Read the model definition and answer for the solid it produces. Units are mm, in the model's axes. A direction names the side the tool comes from. Coordinates: 2 decimals unless noted, no trailing zeros. Write each loop counter-clockwise with the first axis right and the second up, starting at its lowest first coordinate (ties: lowest second). Pieces come first, ordered by that corner, then holes.
1) The part is cut by section A-A (y = 15). Determine the outline of the cut face in (x, z).
2) Each of these flat-tipped pins is pushed along its axis until it touches: pin 1 Ø4 at (x, z) = (1.5, -83.5) entering from -Y; pin 2 Ø4 at (y, z) = (30.5, -4.5) entering from -X. Where does it stop, or does it pass through?
3) Which of the six approach directions +Z, -Z, +X, -X, +Y, -Y give full straight-line access (tool end or side, diameter ignored) to faces 1 (the face through (17, -1, -3)), 2 (the face through (7, 53.5, -3))?
4) Determine the mould class of faces 3 (the face through (15.5, 0, -3)), 4 (the face through (0, 1, -200)), 5 (the face through (0, 1, 200)) for opening direction Z: +Z half, -Z half, draft (parallel to the pull), parting line (faces both ways), or undercut.
5) Find the intervals of material crossed by line 1 (X direction, y = -35, z = 199.2); line 2 (Z direction, x = -2.5, y = 2.5); line 3 (X direction, y = -20, z = 199.2), in increasing order.
6) The part is cut by section B-B (z = 64.5). Determine the outline of the cut face in (x, y), then the cut area to 3 significant figures.
Autodesk Inventor part; units mm, degrees
ref_plane "YZ Plane" through (0, 0, 0) normal (1, 0, 0) x (0, 1, 0)
ref_plane "XZ Plane" through (0, 0, 0) normal (0, 1, 0) x (-1, 0, 0)
ref_plane "XY Plane" through (0, 0, 0) normal (0, 0, 1) x (1, 0, 0)
sketch "Skizze1" plane through (0, 0, 0) normal (0, 0, 1) x (1, 0, 0)
  line L0 (-17, -55) -> (17, -55)
  line L1 (17, -55) -> (17, 55)
  line L2 (17, 55) -> (-17, 55)
  line L3 (-17, 55) -> (-17, -55)
  line L4 (-17, 55) -> (17, -55) construction
  line L5 (-17, -55) -> (17, 55) construction
  point P0 (0, 0)
  point P1 (0, 0)
  dimension "d0" = 34
  dimension "d2" = 110
extrude "Extrusion1" add sketch "Skizze1" along normal mid plane 400
sketch "Skizze2" plane through (0, 0, 200) normal (0, 0, 1) x (1, 0, 0)
  line L0 (-17, -55) -> (17, -55)
  line L1 (17, -55) -> (17, 55)
  line L2 (17, 55) -> (-17, 55)
  point P0 (0, 0)
  point P1 (2, 30)
  point P2 (9, -20)
  point P3 (2, -35)
  dimension "d5" = 25
  dimension "d6" = 15
  dimension "d30" = 50
  dimension "d31" = 8
  dimension "d32" = 7
  dimension "d33" = 35
  dimension "d40" = 20
  dimension "d41" = 15
hole "Bohrung1" at (2, 30, 200) at (9, -20, 200) at (2, -35, 200) direction (0, 0, -1) diameter 4 end through all
sketch "Skizze4" plane through (-17, -55, 200) normal (-1, 0, 0) x (0, 0, 1)
  line L0 (0, 0) -> (-400, 0)
  line L1 (0, 110) -> (0, 0)
  line L2 (-400, 110) -> (0, 110)
  line L3 (-400, 0) -> (-400, 110)
  line L4 (-398.5, 108.5) -> (-1.5, 108.5)
  line L5 (-1.5, 108.5) -> (-1.5, 0)
  line L6 (-1.5, 0) -> (-398.5, 0)
  line L7 (-398.5, 0) -> (-398.5, 108.5)
  point P0 (-200, 55)
  dimension "d34" = 1.5
  dimension "d35" = 0
  dimension "d36" = 1.5
  dimension "d37" = 1.5
extrude "Extrusion2" cut sketch "Skizze4" against normal blind 32.5 contours L0 L7 L4 L5
sketch "Skizze5" plane through (-17, 55, 200) normal (0, 1, 0) x (1, 0, 0)
  line L0 (34, 0) -> (0, 0)
  line L1 (34, 400) -> (34, 0)
  line L2 (0, 400) -> (34, 400)
  line L3 (0, 398.5) -> (16, 398.5)
  line L4 (16, 398.5) -> (16, 1.5)
  line L5 (16, 1.5) -> (0, 1.5)
  line L6 (0, 1.5) -> (0, 398.5)
  point P0 (17, 200)
  dimension "d42" = 1.5
  dimension "d43" = 1.5
  dimension "d44" = 18
extrude "Extrusion3" cut sketch "Skizze5" against normal blind 32.5
properties part number "bewegliche achse horizontal" material "Stahl"
Reported:
1. outline: (-17, -200) - (17, -200) - (17, 200) - (-17, 200) - (-17, 198.5) - (15.5, 198.5) - (15.5, -198.5) - (-17, -198.5) - close
2. pin 1: stops at y = 53.5
2. pin 2: stops at x = 15.5
3. face 1: +Z, -Z, +X, +Y, -Y
3. face 2: -X, -Y
4. face 3: undercut
4. face 4: -Z half
4. face 5: +Z half
5. line 1: x = -17 to 0, 4 to 17
5. line 2: z = -200 to -198.5, 198.5 to 200
5. line 3: x = -17 to 7, 11 to 17
6. outline: (-1, 53.5) - (15.5, 53.5) - (15.5, -55) - (17, -55) - (17, 55) - (-1, 55) - close
6. area: 190 mm2
